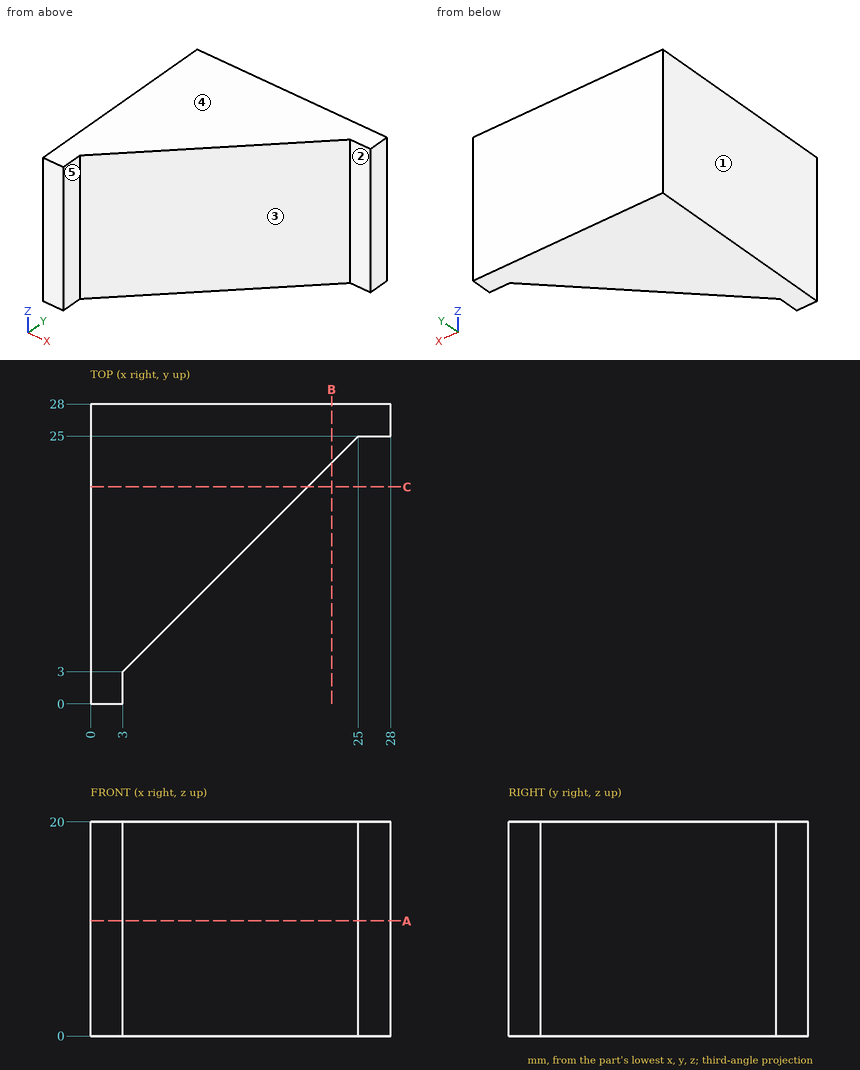
Answer from the drawing. Dimensions are ordinates in mm from the lowest x, y and z of the part. A direction names the side the tool comes from. Coordinates: 2 decimals unless noted, no trailing zeros. Write each loop counter-clockwise with the first axis right and the second up, starting at its lowest first coordinate (ties: lowest second). Pieces come first, ordered by that corner, then holes. Notation, with made-up numbers: (46, 79) - (104, 79) arc R26 cw to (104, 105) - close; hole circle Ø7 at (14, 39). An arc over 180 degrees is marked (long way). Return JSON: item names as keys, results as strings. Group by question number.
Q1. Which of the six approach directions +Z, -Z, +X, -X, +Y, -Y give full straight-line access (tool end or side, diameter ignored) to the marked faces 4 and 5?
Q2. For a pull along X with two mould halves and no side action, classify the marked faces 1, 2 and 3 as +X half, -X half, draft (parallel to the pull), parting line (faces both ways), or undercut.
Q3. Find the intervals of material crossed by line 1 along X through (y, z) = (2.25, 3.25); line 2 along X through (y, z) = (11, 12.5); line 3 along Y through (x, z) = (18, 1), in increasing order. Write a range as [from, to].
Q4. The part is cut by section B-B on x = 22.5. Write down the section's boundary in (y, z).
Q5. Flat-ended cylindrical pins translate along their axes: pin 1 Ø4 at (x, z) = (6, 15.5) entering from -Y; pin 2 Ø3 at (x, y) = (7.5, 6.5) entering from -Z; pin 3 Ø3.5 at (x, z) = (27, 7) entering from -Y; pin 4 Ø5 at (y, z) = (16.5, 9.5) entering from +X. Find the tip coordinate at first contact, or state that the pin passes through.
Q6. The part is cut by section C-C on y = 20.25. Write down the section's boundary in (x, z), and give its area (3 significant figures).
Q7. The part is cut by section A-A on z = 10.75. Write down the section's boundary in (x, y).
Evaluation:
{
 "1": {"face 4": "+Z, +X, -X, +Y, -Y", "face 5": "+Z, -Z, +X, -Y"},
 "2": {"face 1": "-X half", "face 2": "draft", "face 3": "+X half"},
 "3": {"line 1": "x = [0, 3]", "line 2": "x = [0, 11]", "line 3": "y = [18, 28]"},
 "4": {"outline": "(22.5, 0) - (28, 0) - (28, 20) - (22.5, 20) - close"},
 "5": {"pin 1": "stops at y = 4", "pin 2": "stops at z = 0", "pin 3": "stops at y = 25", "pin 4": "stops at x = 19"},
 "6": {"outline": "(0, 0) - (20.25, 0) - (20.25, 20) - (0, 20) - close", "area": "405 mm2"},
 "7": {"outline": "(0, 0) - (3, 0) - (3, 3) - (25, 25) - (28, 25) - (28, 28) - (0, 28) - close"}
}
